Build history of the part. All positions in model axes, mm. A direction names the side the tool comes from. Give positions to 0.01 mm unless a question says otherwise; leave off trailing zeros. Loops run counter-clockwise (first coordinate to the right, second up) from the corner with the lowest first, then second, coordinate; pieces in that order, holes last. Notation, with made-up numbers: M 25,23.25 L 76,23.25 A19 cw 76,50.25 Z; hole C 55.25,9 d10. An arc over 180 degrees is marked long. Put each result on its own line as item: value.
```python
from build123d import *

# Parameters (mm, degrees)
F0_R     = 18.75
F0_R_2   = 13.75
F1_DEPTH = 40
F3_DEPTH = 30
F4_R     = 1.6
F5_DEPTH = 19.750000113
F6_DEPTH = 16.75
F8_R     = 2.5
F9_DEPTH = 5
F10_R    = 4.99999


# Not quite as in the source:
# - a fillet or chamfer is up to 0.001 mm smaller than in the source, because OpenCascade refuses the exact size


with BuildPart() as f1:
    # F0 (on Front) → F1 (new body)
    with BuildSketch(Plane.XZ):
        Circle(F0_R)
        Circle(F0_R_2, mode=Mode.SUBTRACT)
    extrude(amount=F1_DEPTH)

    # F2 (on face) → F3 (cut)
    with BuildSketch(Plane.XZ.offset(40)):
        with BuildLine():
            ThreePointArc((-11, 8.25), (0, 13.75), (11, 8.25))
            Line((11, 8.25), (15, 11.25))
            ThreePointArc((15, 11.25), (0, 18.75), (-15, 11.25))
            Line((-15, 11.25), (-11, 8.25))
        make_face()
        with BuildLine():
            Line((15, -11.25), (11, -8.25))
            ThreePointArc((11, -8.25), (0, -13.75), (-11, -8.25))
            Line((-11, -8.25), (-15, -11.25))
            ThreePointArc((-15, -11.25), (0, -18.75), (15, -11.25))
        make_face()
    extrude(amount=-F3_DEPTH, mode=Mode.SUBTRACT)

    # F4 (on Right) → F5 (cut, up to face)
    with BuildSketch(Plane.YZ):
        with Locations((-20, 0)):
            Circle(F4_R)
    extrude(amount=-F5_DEPTH, mode=Mode.SUBTRACT)

    # F4 (on Right) → F6 (cut)
    with BuildSketch(Plane.YZ):
        Polygon((-22.9, 1.6743157806), (-22.9, -1.6743157806), (-20, -3.3486315613), (-17.1, -1.6743157806), (-17.1, 1.6743157806), (-20, 3.3486315613), align=None)
        with Locations((-20, 0)):
            Circle(F4_R, mode=Mode.SUBTRACT)
    extrude(amount=-F6_DEPTH, mode=Mode.SUBTRACT)

    # F8 (on offset) → F9 (join)
    with BuildSketch(Plane.YZ.offset(20)):
        Polygon((0, 11.25), (-60, 11.25), (-60, 15), (-75, 15), (-75, -15), (-60, -15), (-60, -11.25), (0, -11.25), align=None)
        with Locations((-67.5, -10)):
            Circle(F8_R, mode=Mode.SUBTRACT)
        with Locations((-67.5, 0)):
            Circle(F8_R, mode=Mode.SUBTRACT)
        with Locations((-52.5, 0)):
            Circle(F8_R, mode=Mode.SUBTRACT)
        with Locations((-67.5, 10)):
            Circle(F8_R, mode=Mode.SUBTRACT)
    extrude(amount=-F9_DEPTH)

    # F10 (radius 5 in the source; OpenCascade refuses exactly that, so slightly less here)
    f10_edges = [f1.edges().sort_by_distance(p)[0] for p in [
        (20, -30, 11.25),
        (20, -30, -11.25),
    ]]
    fillet(f10_edges, radius=F10_R)


solid = f1.part
```
Q1. Mould opens along Z. For faces 1 (the flat face through (18, -75, 0)), 2 (the flat face through (18, -68, -15)), 3 (the cylindrical face through (18.5, -30.42, 9.82)), 4 (the cylindrical face through (-17.74, -21.18, 1.08)) say: pulls with the +Z half, pulls with the -Z half, needs draft (parallel to the pull), parting line crosses it, or undercut.
Here are the results:
face 1: needs draft
face 2: pulls with the -Z half
face 3: pulls with the +Z half
face 4: undercut
Q2. Drop flat-ended pins along their axis: pin 1 Ø3 at (x, z) = (7, 11.5) entering from -Y; pin 2 Ø2.5 at (x, y) = (18.5, -66.5) entering from -Z; pin 3 Ø12 at (x, y) = (7, -9.5) entering from +Z; pin 4 Ø2 at (x, y) = (9, -28) entering from +Z. Give the stop position or say it passes through.
Here are the results:
pin 1: y = -10
pin 2: z = -15
pin 3: z = 18.72
pin 4: through
Q3. Probe line 1 (Z direction, x = 18.7, y = -67.5); line 2 (Y direction, x = -18.05, z = 0); line 3 (Y direction, x = -15.5, z = -1). List the from-to ranges inside material, lowest first. Write a range as from..to.
Here are the results:
line 1: -15..-12.5, -7.5..-2.5, 2.5..7.5, 12.5..15
line 2: -40..-21.6, -18.4..0
line 3: -40..-22.9, -17.1..0
Q4. Slice it at A-A (z = 0). List the corners of the cut face in (x, y).
Here are the results:
outline: M -18.75,-40 L -13.75,-40 L -13.75,-22.9 L -16.75,-22.9 L -16.75,-21.6 L -18.75,-21.6 Z; M -18.75,-18.4 L -16.75,-18.4 L -16.75,-17.1 L -13.75,-17.1 L -13.75,0 L -18.75,0 Z; M 13.75,-40 L 15,-40 L 15,-50 L 20,-50 L 20,0 L 13.75,0 Z; M 15,-75 L 20,-75 L 20,-70 L 15,-70 Z; M 15,-65 L 20,-65 L 20,-55 L 15,-55 Z
Q5. Tool access for faces 5 (the cylindrical face through (18.57, -29.58, -9.75)), 6 (the flat face through (0, -10, 15)), 7 (the flat face through (-16.75, -19, 2)): list every direction of +Z, -Z, +X, -X, +Y, -Y with a clear straight run to the whole face (end or side of a thin tool).
Here are the results:
face 5: -Z, +X, +Y
face 6: +Z, -Y
face 7: none
Q6. Slice it at C-C (x = -2). List the corners of the cut face in (y, z), and give its area (3 significant figures).
Here are the results:
outline: M -10,-18.64 L 0,-18.64 L 0,-13.6 L -10,-13.6 Z; M -10,13.6 L 0,13.6 L 0,18.64 L -10,18.64 Z
area: 101 mm²
Q7. Slice it at D-D (z = 10). List the corners of the cut face in (x, y).
Here are the results:
outline: M -15.86,-40 L -13.33,-40 L -13.33,-10 L -9.44,-10 L -9.44,0 L -15.86,0 Z; M 9.44,-10 L 13.33,-10 L 13.33,-40 L 15,-40 L 15,-65 L 20,-65 L 20,-60 L 18.31,-60 L 18.31,0 L 9.44,0 Z; M 15,-75 L 20,-75 L 20,-70 L 15,-70 Z
